Source: CAD feature listing. Evaluate the final solid. Frame: model axes, mm. Face numbers are marked on the shaded views. Coordinates: 2 decimals unless noted, no trailing zeros. Write each loop counter-clockwise with the first axis right and the second up, starting at its lowest first coordinate (ties: lowest second). Pieces come first, ordered by that corner, then holes. Notation, with made-up numbers: (54, 61.5) - (105, 61.5) arc R18 ccw to (105, 83.5) - close; hole circle Ø5 at (14, 55). An arc over 180 degrees is marked (long way). One line per item, written item: value.
from build123d import *

# Parameters (mm, degrees)
EXTRUDE_1_DEPTH     = 2
SKETCH_2_R          = 2.75
SKETCH_2_R_2        = 1.1
SKETCH_2_R_3        = 0.6
CUT_EXTRUDE_1_DEPTH = 2


with BuildPart() as part:
    # 草图1 → 凸台-拉伸1 (new body)
    with BuildSketch(Plane.XY):
        with BuildLine():
            Line((-16.234375, 2.488989425), (-0.375, 3.982383081))
            ThreePointArc((-0.375, 3.982383081), (0, 4), (0.375, 3.982383081))
            Line((0.375, 3.982383081), (16.234375, 2.488989425))
            ThreePointArc((16.234375, 2.488989425), (18.5, 0), (16.234375, -2.488989425))
            Line((16.234375, -2.488989425), (0.375, -3.982383081))
            ThreePointArc((0.375, -3.982383081), (0, -4), (-0.375, -3.982383081))
            Line((-0.375, -3.982383081), (-16.234375, -2.488989425))
            ThreePointArc((-16.234375, -2.488989425), (-18.5, 0), (-16.234375, 2.488989425))
        make_face()
    extrude(amount=EXTRUDE_1_DEPTH)

    # 草图2 → 切除-拉伸1 (cut)
    with BuildSketch(Plane.XY.offset(2)):
        Circle(SKETCH_2_R)
        with Locations((-16, 0)):
            Circle(SKETCH_2_R_2)
        with Locations((16, 0)):
            Circle(SKETCH_2_R_2)
        with Locations((-4.5, 0)):
            Circle(SKETCH_2_R_3)
        with Locations((-6.5, 0)):
            Circle(SKETCH_2_R_3)
        with Locations((-8.5, 0)):
            Circle(SKETCH_2_R_3)
        with Locations((-10.5, 0)):
            Circle(SKETCH_2_R_3)
        with Locations((4.5, 0)):
            Circle(SKETCH_2_R_3)
        with Locations((10.5, 0)):
            Circle(SKETCH_2_R_3)
        with Locations((8.5, 0)):
            Circle(SKETCH_2_R_3)
        with Locations((6.5, 0)):
            Circle(SKETCH_2_R_3)
    extrude(amount=-CUT_EXTRUDE_1_DEPTH, mode=Mode.SUBTRACT)


solid = part.part
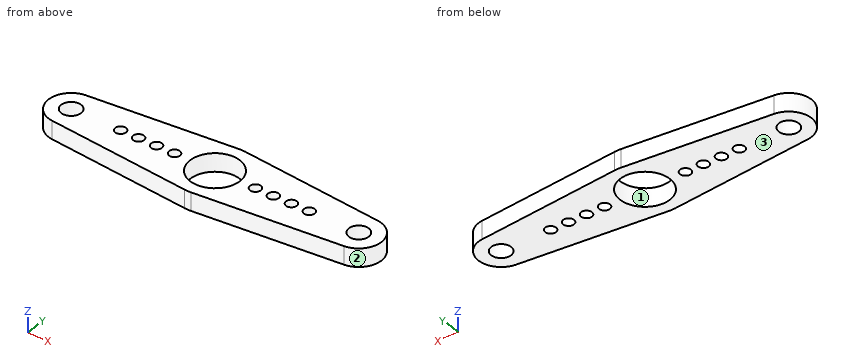
1) Draft query along X for the marked faces 1, 2 and 3. Return one class per face: released by +X, released by -X, zero draft, split by the parting line, or undercut.
Values found:
face 1: undercut
face 2: released by +X
face 3: zero draft
2) Section query C-C on z = 0.55. State how many separate pieces and enclosed holes the cut face has, then the cut area to 3 significant figures.
Values found:
separate pieces: 1
enclosed holes: 11
area: 188 mm2
3) Material intervals for line 1 (X direction, y = -1, z = 1.95); line 2 (X direction, y = 2, z = 0.85); line 3 (Y direction, x = -0.5, z = 1.05), sorted ascending.
Values found:
line 1: -18.29 to -16.46, -15.54 to -2.56, 2.56 to 15.54, 16.46 to 18.29
line 2: -17.5 to -1.89, 1.89 to 17.5
line 3: -3.97 to -2.7, 2.7 to 3.97
4) Section query B-B on y = -1.5. Output: boundary loops of the cut face in (x, z).
Values found:
outline: (-18, 0) - (-2.3, 0) - (-2.3, 2) - (-18, 2) - close; (2.3, 0) - (18, 0) - (18, 2) - (2.3, 2) - close
5) Contact query for flat-ended pins moving along their axis: P1, Ø1, axis at y = -1, z = 1, coming from the +X side; P2, Ø1, axis at x = -13, z = 1.5, coming from the -Y side. Output: stop coordinate, or through.
Values found:
P1: x = 18.45
P2: y = -2.84
6) Section query A-A on x = 0. Output: boundary loops of the cut face in (y, z), then the cut area to 3 significant figures.
Values found:
outline: (-4, 0) - (-2.75, 0) - (-2.75, 2) - (-4, 2) - close; (2.75, 0) - (4, 0) - (4, 2) - (2.75, 2) - close
area: 5.00 mm2
